from build123d import *

# Parameters (mm, degrees)
F0_R      = 7.5
F0_R_2    = 6.5
F1_DEPTH  = 10
F2_R      = 9
F2_R_2    = 7.5
F3_DEPTH  = 1.5
F4_SIZE   = 1
F5_R      = 9
F5_R_2    = 7.5
F6_DEPTH  = 1.5
F7_SIZE   = 1
F6_FACE_R = 6.5
F8_DEPTH  = 25
F9_R      = 0.5
F10_R     = 0.5


with BuildPart() as f1:
    # F0 (on Top) → F1 (new body)
    with BuildSketch(Plane.XY):
        Circle(F0_R)
        Circle(F0_R_2, mode=Mode.SUBTRACT)
    extrude(amount=F1_DEPTH)

    # F2 (on face) → F3 (join)
    with BuildSketch(Plane.XY.offset(10)):
        Circle(F2_R)
        Circle(F2_R_2, mode=Mode.SUBTRACT)
    extrude(amount=-F3_DEPTH)

    # F4
    f4_edges = [f1.edges().sort_by_distance(p)[0] for p in [
        (-9, 0, 8.5),
    ]]
    chamfer(f4_edges, length=F4_SIZE)

    # F5 (on face) → F6 (join)
    with BuildSketch(Plane(origin=(0, 0, 0), x_dir=(1, 0, 0), z_dir=(0, 0, -1))):
        Circle(F5_R)
        Circle(F5_R)
        Circle(F5_R_2, mode=Mode.SUBTRACT)
    extrude(amount=-F6_DEPTH)

    # F7
    f7_edges = [f1.edges().sort_by_distance(p)[0] for p in [
        (-9, 0, 1.5),
    ]]
    chamfer(f7_edges, length=F7_SIZE)

    # F6_face (on face) → F8 (cut)
    with BuildSketch(Plane.XY.offset(1.5)):
        Circle(F6_FACE_R)
    extrude(amount=-F8_DEPTH, mode=Mode.SUBTRACT)

    # F9
    f9_edges = [f1.edges().sort_by_distance(p)[0] for p in [
        (-6.5, 0, 0),
    ]]
    fillet(f9_edges, radius=F9_R)

    # F10
    f10_edges = [f1.edges().sort_by_distance(p)[0] for p in [
        (-6.5, 0, 10),
    ]]
    fillet(f10_edges, radius=F10_R)


solid = f1.part
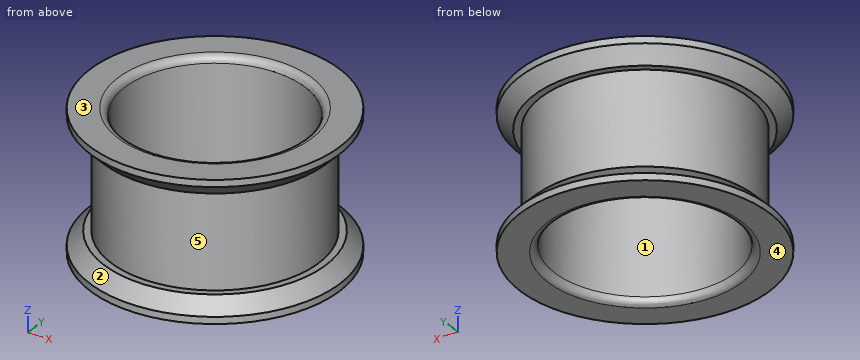
Can you work these out from the model? Positions are in its coordinate system, mm. Face numbers are marked on the shaded views. A direction names the side the tool comes from. Round coordinates to 2 decimals unless told otherwise and drop trailing zeros. Write each loop counter-clockwise with the first axis right and the second up, starting at its lowest first coordinate (ties: lowest second). Pieces come first, ordered by that corner, then holes. Notation, with made-up numbers: M -3,-18.5 L 22,-18.5 A12 ccw 22,-10.5 Z; hole C 55,63 d4. An arc over 180 degrees is marked long. Use a Markdown table: item, result.
Item 1: For pin 1 Ø6 at (y, z) = (-3, 7.5) entering from +X; pin 2 Ø1 at (x, y) = (-1, 4) entering from +Z; pin 3 Ø6 at (x, z) = (-3.5, 7) entering from +Y, each with a flat end and sliding along its axis, tell me the tip position at first contact or that it passes through.
Found:
| item | result |
|---|---|
| pin 1 | stops at x = 8.97 |
| pin 2 | passes through |
| pin 3 | stops at y = 8.81 |
Item 2: Which directions (+Z, -Z, +X, -X, +Y, -Y) give clear straight access to the entire face, cutting with the end or side of a thin tool? Please do the marked faces 4 and 5.
Found:
| item | result |
|---|---|
| face 4 | -Z, +X, -X, +Y, -Y |
| face 5 | none |
Item 3: We'd pull the mould along Z, two halves only. Please class the marked faces 1, 2 and 3: released by +Z, released by -Z, zero draft, split by the parting line, or undercut.
Found:
| item | result |
|---|---|
| face 1 | zero draft |
| face 2 | undercut |
| face 3 | released by +Z |
Item 4: I want a section at A-A (x = 0). List the corners of the cut face in (y, z) for me, and give its area (3 significant figures).
Found:
| item | result |
|---|---|
| outline | M -9,0 L -7,0 A0.5 ccw -6.5,0.5 L -6.5,9.5 A0.5 ccw -7,10 L -9,10 L -9,9.5 L -8,8.5 L -7.5,8.5 L -7.5,1.5 L -8,1.5 L -9,0.5 Z; M 6.5,0.5 A0.5 ccw 7,0 L 9,0 L 9,0.5 L 8,1.5 L 7.5,1.5 L 7.5,8.5 L 8,8.5 L 9,9.5 L 9,10 L 7,10 A0.5 ccw 6.5,9.5 Z |
| area | 26.8 mm2 |
Item 5: I want a section at C-C (z = 3). List the corners of the cut face in (x, y) for me.
Found:
| item | result |
|---|---|
| outline | C 0,0 d15; hole C 0,0 d13 |
Item 6: If I drill on line 1 along Y through (x, z) = (0, 6.25); line 2 along X through (y, z) = (1.75, 4.5), over which ranges is the centre line in solid material (lowest first)? Write a range as [from, to].
Found:
| item | result |
|---|---|
| line 1 | y = [-7.5, -6.5], [6.5, 7.5] |
| line 2 | x = [-7.29, -6.26], [6.26, 7.29] |
